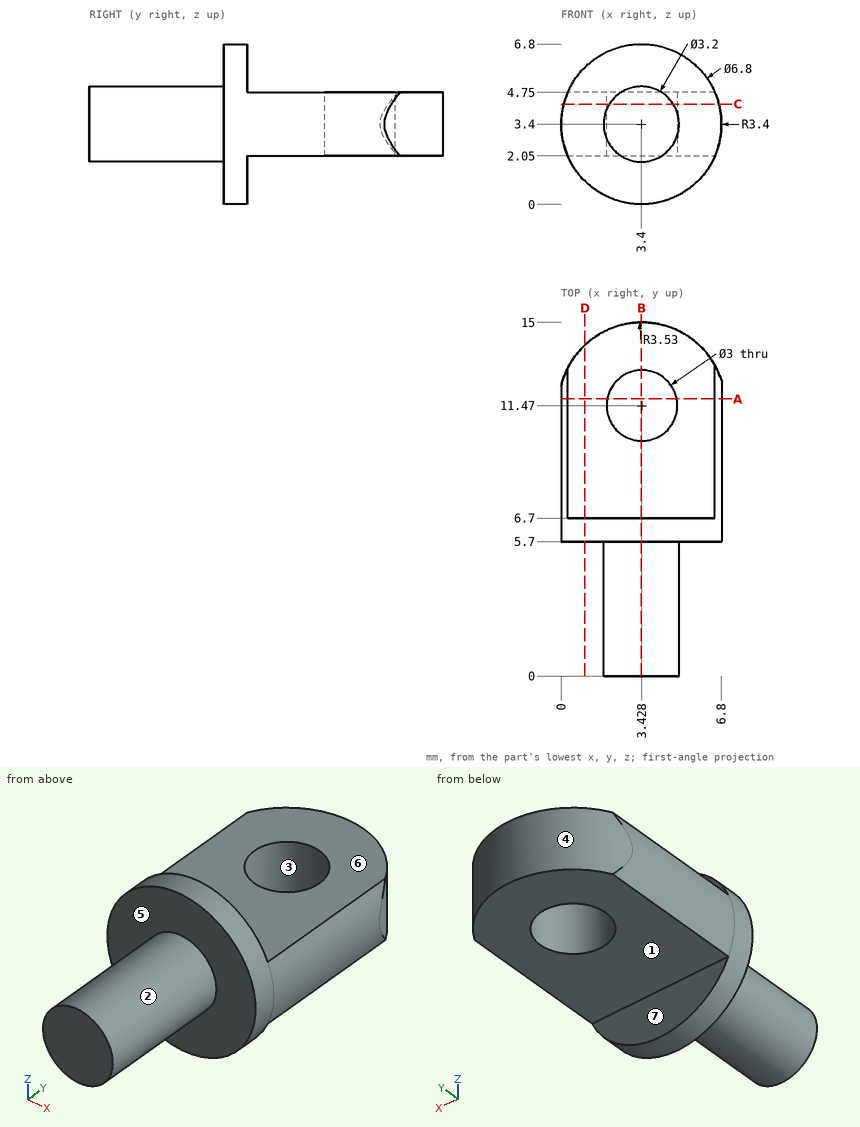
Geometry check sheet. Reference: drawing and pictorial views, mm from the part's lowest x, y, z. A direction names the side the tool comes from. Give positions to 0.01 mm unless a question says otherwise; leave off trailing zeros. Write each loop counter-clockwise with the first axis right and the second up, starting at its lowest first coordinate (ties: lowest second). Pieces come first, ordered by that corner, then holes. Notation, with made-up numbers: (17, 61) - (48, 61) arc R34 ccw to (48, 91) - close; hole circle Ø7 at (-33, 87). An arc over 180 degrees is marked (long way). Use a Markdown table: item, result.
Q1. Section check B-B, the plane x = 3.4. Enter the section's corners in (y, z).
Computed:
| item | result |
|---|---|
| outline | (0, 1.8) - (5.7, 1.8) - (5.7, 0) - (6.7, 0) - (6.7, 2.05) - (9.97, 2.05) - (9.97, 4.75) - (6.7, 4.75) - (6.7, 6.8) - (5.7, 6.8) - (5.7, 5) - (0, 5) - close; (12.97, 2.05) - (15, 2.05) - (15, 4.75) - (12.97, 4.75) - close |
Q2. Section check A-A, the plane y = 11.75. Enter the section's corners in (x, z).
Computed:
| item | result |
|---|---|
| outline | (0.28, 2.05) - (1.95, 2.05) - (1.95, 4.75) - (0.28, 4.75) arc R3.4 ccw to start; (4.9, 2.05) - (6.52, 2.05) arc R3.4 ccw to (6.52, 4.75) - (4.9, 4.75) - close |
Q3. Draft check along X on the marked faces 1, 2 and 3. Enter one of: pulls with the +X half, pulls with the -X half, needs draft (parallel to the pull), parting line crosses it, or undercut.
Computed:
| item | result |
|---|---|
| face 1 | needs draft |
| face 2 | parting line crosses it |
| face 3 | undercut |
Q4. Go/stop test with flat-tipped pins: P1, Ø1, axis at x = 2.5, z = 1, coming from the +Y side; P2, Ø2, axis at x = 2, z = 3, coming from the -Y side; P3, Ø2.5, axis at x = 3.43, y = 11.47, coming from the +Z side; P4, Ø1, axis at y = 2, z = 2, coming from the -X side. Record where each tip stops, or that it passes through.
Computed:
| item | result |
|---|---|
| P1 | stops at y = 6.7 |
| P2 | stops at y = 0 |
| P3 | passes through |
| P4 | stops at x = 2.08 |
Q5. Section check C-C, the plane z = 4.25. Enter the section's corners in (x, y), then the cut area to 3 significant figures.
Computed:
| item | result |
|---|---|
| outline | (0.11, 5.7) - (2.04, 5.7) - (2.04, 0) - (4.76, 0) - (4.76, 5.7) - (6.69, 5.7) - (6.69, 12.81) arc R3.53 ccw to (0.11, 12.67) - close; hole circle Ø3 at (3.43, 11.47) |
| area | 65.5 mm² |
Q6. Set-up check for the marked faces 4, 5, 6 and 7: record each of +Z, -Z, +X, -X, +Y, -Y from which the full face is reachable in a straight line by a thin tool's end or side.
Computed:
| item | result |
|---|---|
| face 4 | +Z, -Z, +Y |
| face 5 | -Y |
| face 6 | +Z, +X, -X, +Y |
| face 7 | -Z, +X, -X, +Y |
Q7. Thickness scan on L1, parallel to Z at x = 3.5, y = 7.75; L2, parallel to Y at x = 4, z = 5.75; L3, parallel to X at y = 11, z = 2.25. Record the ranges inside material, lowest first. Write a range as [from, to].
Computed:
| item | result |
|---|---|
| L1 | z = [2.05, 4.75] |
| L2 | y = [5.7, 6.7] |
| L3 | x = [0.2, 2], [4.85, 6.6] |
Q8. Section check D-D, the plane x = 1. Enter the section's corners in (y, z).
Computed:
| item | result |
|---|---|
| outline | (5.7, 0.99) - (6.7, 0.99) - (6.7, 2.05) - (14.03, 2.05) - (14.03, 4.75) - (6.7, 4.75) - (6.7, 5.81) - (5.7, 5.81) - close |
